Geometry check sheet. Reference: the model listing, model coordinates, mm. A direction names the side the tool comes from. Give positions to 0.01 mm unless a question says otherwise; leave off trailing zeros. Order: outer loops, then holes, each group sorted by start corner. A loop starts at its lowest first (then second) coordinate and runs counter-clockwise, first axis right, second up.
Autodesk Inventor part; units mm, degrees
ref_plane "YZ Plane" through (0, 0, 0) normal (1, 0, 0) x (0, 1, 0)
ref_plane "XZ Plane" through (0, 0, 0) normal (0, 1, 0) x (-1, 0, 0)
ref_plane "XY Plane" through (0, 0, 0) normal (0, 0, 1) x (1, 0, 0)
sketch "Sketch1" plane through (0, 0, 0) normal (0, 0, 1) x (1, 0, 0)
  line L0 (0, 0) -> (119.38, 0)
  line L1 (119.38, 0) -> (119.38, 91.44)
  line L2 (119.38, 91.44) -> (0, 91.44)
  line L3 (0, 91.44) -> (0, 0)
  dimension "d0" = 119.38
  dimension "d1" = 91.44
extrude "Extrusion1" add sketch "Sketch1" along normal blind 27.94
chamfer "Chamfer1" distance 1.27 angle 45 1 edges at (59.69, 0, 0)
chamfer "Chamfer2" distance 1.27 angle 45 1 edges at (0, 46.355, 0)
chamfer "Chamfer3" distance 1.27 angle 45 1 edges at (60.325, 91.44, 0)
chamfer "Chamfer4" distance 1.27 angle 45 1 edges at (119.38, 45.72, 0)
chamfer "Chamfer5" distance 1.27 angle 45 1 edges at (0, 45.72, 27.94)
chamfer "Chamfer6" distance 1.27 angle 45 1 edges at (60.325, 0, 27.94)
chamfer "Chamfer7" distance 1.27 angle 45 2 edges at (60.325, 91.44, 27.94) (119.38, 46.355, 27.94)
sketch "Sketch2" plane through (119.38, 0, 1.27) normal (1, 0, 0) x (0, 0, -1)
  line L0 (-25.4, 0) -> (-25.4, 91.44)
  line L1 (0, 0) -> (-25.4, 0)
  line L2 (-19.05, 0) -> (-19.05, 60.96)
  line L3 (-6.35, 0) -> (-6.35, 60.96)
  line L4 (-19.05, 0) -> (-6.35, 0)
  line L5 (-19.05, 60.96) -> (-22.86, 91.44)
  line L6 (0, 91.44) -> (-25.4, 91.44)
  line L7 (-6.35, 60.96) -> (-2.54, 91.44)
  line L8 (-22.86, 91.44) -> (-2.54, 91.44)
  dimension "d25" = 60.96
  dimension "d26" = 60.96
  dimension "d27" = 12.7
  dimension "d28" = 6.35
  dimension "d29" = 20.32
  dimension "d30" = 2.54
extrude "Extrusion2" add sketch "Sketch2" along normal blind 2.54 contours L2 L5 L6 L7 L3 L1
sketch "Sketch3" plane through (0, 0, 1.27) normal (0, -1, 0) x (1, 0, 0)
  line L0 (0, 0) -> (0, 25.4)
  line L1 (119.38, 19.05) -> (0, 19.05)
  line L2 (119.38, 6.35) -> (0, 6.35)
  line L3 (0, 19.05) -> (0, 6.35)
  line L4 (119.38, 19.05) -> (119.38, 6.35)
extrude "Extrusion3" add sketch "Sketch3" along normal blind 2.54
sketch "Sketch4" plane through (0, 0, 1.27) normal (-1, 0, 0) x (0, 0, 1)
  line L0 (25.4, 91.44) -> (25.4, 0)
  line L1 (0, 91.44) -> (25.4, 91.44)
  line L2 (0, 0) -> (0, 91.44)
  line L3 (0, 0) -> (6.35, 0)
  line L4 (6.35, 0) -> (6.35, -2.54)
  line L5 (19.05, -2.54) -> (6.35, -2.54)
  line L6 (19.05, 0) -> (19.05, -2.54)
  line L7 (19.05, 0) -> (25.4, 0)
sketch "Sketch5" plane through (121.92, 0, 1.27) normal (1, 0, 0) x (0, 0, -1)
  line L0 (-2.54, 91.44) -> (-22.86, 91.44)
  line L1 (-22.86, 91.44) -> (-19.05, 60.96)
  line L2 (-19.05, 60.96) -> (-19.05, 0)
  line L3 (-19.05, 0) -> (-6.35, 0)
  line L4 (-6.35, 0) -> (-6.35, 60.96)
  line L5 (-6.35, 60.96) -> (-2.54, 91.44)
sketch "Sketch6" plane through (0, 0, 1.27) normal (-1, 0, 0) x (0, 0, 1)
  line L0 (25.4, 91.44) -> (25.4, 0)
  line L1 (0, 91.44) -> (25.4, 91.44)
  line L2 (19.05, -2.54) -> (6.35, -2.54)
  line L3 (6.35, 0) -> (6.35, 60.96)
  line L4 (6.35, 0) -> (6.35, 60.96)
  line L5 (19.05, 60.96) -> (19.05, 0)
  line L6 (19.05, 0) -> (6.35, 0)
  line L7 (6.35, 60.96) -> (2.54, 91.44)
  line L8 (2.54, 91.44) -> (6.35, 60.96)
  line L9 (19.05, 60.96) -> (22.86, 91.44)
  line L10 (2.54, 91.44) -> (22.86, 91.44)
  dimension "d35" = 60.96
  dimension "d36" = 2.54
  dimension "d37" = 6.35
extrude "Extrusion4" add sketch "Sketch6" along normal blind 2.54
sketch "Sketch7" plane through (0, 0, 27.94) normal (0, 0, 1) x (1, 0, 0)
  line L0 (1.27, 90.17) -> (118.11, 90.17)
  line L1 (20.32, 82.55) -> (20.32, 74.93)
  line L2 (20.32, 74.93) -> (21.59, 74.93)
  line L3 (21.59, 74.93) -> (21.59, 82.55)
  line L4 (21.59, 82.55) -> (20.32, 82.55)
  line L5 (0, 91.44) -> (0, 0)
  line L6 (26.67, 82.55) -> (26.67, 74.93)
  line L7 (26.67, 74.93) -> (27.94, 74.93)
  line L8 (27.94, 74.93) -> (27.94, 82.55)
  line L9 (27.94, 82.55) -> (26.67, 82.55)
  line L10 (33.02, 82.55) -> (33.02, 74.93)
  line L11 (33.02, 74.93) -> (34.29, 74.93)
  line L12 (34.29, 74.93) -> (34.29, 82.55)
  line L13 (34.29, 82.55) -> (33.02, 82.55)
  line L14 (39.37, 82.55) -> (39.37, 74.93)
  line L15 (39.37, 74.93) -> (40.64, 74.93)
  line L16 (40.64, 74.93) -> (40.64, 82.55)
  line L17 (40.64, 82.55) -> (39.37, 82.55)
  line L18 (45.72, 82.55) -> (45.72, 74.93)
  line L19 (45.72, 74.93) -> (46.99, 74.93)
  line L20 (46.99, 74.93) -> (46.99, 82.55)
  line L21 (46.99, 82.55) -> (45.72, 82.55)
  line L22 (52.07, 82.55) -> (52.07, 74.93)
  line L23 (52.07, 74.93) -> (53.34, 74.93)
  line L24 (53.34, 74.93) -> (53.34, 82.55)
  line L25 (53.34, 82.55) -> (52.07, 82.55)
  line L26 (58.42, 82.55) -> (58.42, 74.93)
  line L27 (58.42, 74.93) -> (59.69, 74.93)
  line L28 (59.69, 74.93) -> (59.69, 82.55)
  line L29 (59.69, 82.55) -> (58.42, 82.55)
  line L30 (64.77, 82.55) -> (64.77, 74.93)
  line L31 (64.77, 74.93) -> (66.04, 74.93)
  line L32 (66.04, 74.93) -> (66.04, 82.55)
  line L33 (66.04, 82.55) -> (64.77, 82.55)
  line L34 (71.12, 82.55) -> (71.12, 74.93)
  line L35 (71.12, 74.93) -> (72.39, 74.93)
  line L36 (72.39, 74.93) -> (72.39, 82.55)
  line L37 (72.39, 82.55) -> (71.12, 82.55)
  line L38 (77.47, 82.55) -> (77.47, 74.93)
  line L39 (77.47, 74.93) -> (78.74, 74.93)
  line L40 (78.74, 74.93) -> (78.74, 82.55)
  line L41 (78.74, 82.55) -> (77.47, 82.55)
  line L42 (83.82, 82.55) -> (83.82, 74.93)
  line L43 (83.82, 74.93) -> (85.09, 74.93)
  line L44 (85.09, 74.93) -> (85.09, 82.55)
  line L45 (85.09, 82.55) -> (83.82, 82.55)
  line L46 (90.17, 82.55) -> (90.17, 74.93)
  line L47 (90.17, 74.93) -> (91.44, 74.93)
  line L48 (91.44, 74.93) -> (91.44, 82.55)
  line L49 (91.44, 82.55) -> (90.17, 82.55)
  line L50 (96.52, 82.55) -> (96.52, 74.93)
  line L51 (96.52, 74.93) -> (97.79, 74.93)
  line L52 (97.79, 74.93) -> (97.79, 82.55)
  line L53 (97.79, 82.55) -> (96.52, 82.55)
  dimension "d40" = 7.62
  dimension "d41" = 1.27
  dimension "d42" = 7.62
  dimension "d44" = 20.32
  dimension "d47" = 6.35
extrude "Extrusion5" cut sketch "Sketch7" against normal blind 3.175
properties part number "Wireless Router"
Q1. Gauge pin test, flat ends, axial feed: P1, Ø2.5, axis at y = 78.5, z = 26.5, coming from the -X side; P2, Ø1.6, axis at y = 77, z = 26, coming from the +X side; P3, Ø2, axis at x = 120.5, y = 41.5, coming from the +Z side. Record the tip position at first contact, or that the pin passes through.
Q2. Cross-section at C-C, the plane y = 71. Record the boundary of the cut face in (x, z) (3 decimals).
Q3. Access from +Z, -Z, +X, -X, +Y, -Y to the whole of each face (thin tool, end or side, straight path). Record for faces 1 (the face through (61, -1, 20.32)), 2 (the face through (-1.3, 76, 22.2)), 3 (the face through (121, 0, 14)), 4 (the face through (-1.25, 75.99, 5.74)), 5 (the face through (85.09, 79, 26)).
Q4. Cross-section at A-A, the plane x = 56.5. Record the boundary of the cut face in (y, z), and give its area (3 significant figures).
Q5. Cross-section at D-D, the plane y = 10. Record the boundary of the cut face in (x, z), and give its area (3 significant figures).
Q6. Cross-section at B-B, the plane z = 6. Record the boundary of the cut face in (x, y).
Q7. Thickness scan on L1, parallel to Y at x = 53, z = 25.25; L2, parallel to Y at x = 93, z = 25.5; L3, parallel to X at y = 59.5, z = 2. Record the ranges inside material, lowest first.
Q8. Release check for a two-part mould opening along Z. For faces 6 (the face through (66.04, 79, 26)), 7 (the face through (59, 46, 27.94)), 8 (the face through (120.63, 75.99, 5.74)) record: pulls with the +Z half, pulls with the -Z half, needs draft (parallel to the pull), parting line crosses it, or undercut.
Answers follow:
1. P1: stops at x = 0
1. P2: stops at x = 119.38
1. P3: stops at z = 20.32
2. outline: (-2.54, 6.365) - (0, 6.365) - (0, 1.27) - (1.27, 0) - (118.11, 0) - (119.38, 1.27) - (119.38, 6.365) - (121.92, 6.365) - (121.92, 21.575) - (119.38, 21.575) - (119.38, 26.67) - (118.11, 27.94) - (1.27, 27.94) - (0, 26.67) - (0, 21.575) - (-2.54, 21.575) - close
3. face 1: +Z, +X, -X, -Y
3. face 2: +Z, -X, -Y
3. face 3: +Z, -Z, +X, -Y
3. face 4: -Z, -X, -Y
3. face 5: +Z
4. outline: (-2.54, 7.62) - (0, 7.62) - (0, 1.27) - (1.27, 0) - (90.17, 0) - (91.44, 1.27) - (91.44, 26.67) - (90.17, 27.94) - (1.27, 27.94) - (0, 26.67) - (0, 20.32) - (-2.54, 20.32) - close
4. area: 2,580 mm2
5. outline: (-2.54, 7.62) - (0, 7.62) - (0, 1.27) - (1.27, 0) - (118.11, 0) - (119.38, 1.27) - (119.38, 7.62) - (121.92, 7.62) - (121.92, 20.32) - (119.38, 20.32) - (119.38, 26.67) - (118.11, 27.94) - (1.27, 27.94) - (0, 26.67) - (0, 20.32) - (-2.54, 20.32) - close
5. area: 3,400 mm2
6. outline: (-2.54, 73.92) - (0, 73.92) - (0, 0) - (119.38, 0) - (119.38, 73.92) - (121.92, 73.92) - (121.92, 91.44) - (-2.54, 91.44) - close
7. L1: y = 0 to 74.93, 82.55 to 91.44
7. L2: y = 0 to 91.44
7. L3: x = 0 to 119.38
8. face 6: needs draft
8. face 7: pulls with the +Z half
8. face 8: pulls with the -Z half
